from build123d import *

# Parameters (mm, degrees)
F1_DEPTH       = 110
F2_R           = 2
F4_D           = 8
F4_DEPTH       = 4
F6_D           = 4
F6_DEPTH       = 4
F6_CSINK_D     = 8
F6_CSINK_ANGLE = 90
F7_W           = 30
F7_H           = 13
F8_DEPTH       = 1


with BuildPart() as f1:
    # F0 (on Top) → F1 (new body)
    with BuildSketch(Plane.XY):
        Polygon((15, -18.36), (15, -15), (-15, -15), (-15, 15), (15, 15), (15, 18.36), (-18.36, 18.36), (-18.36, -18.36), align=None)
    extrude(amount=F1_DEPTH)

    # F2
    f2_edges = [f1.edges().sort_by_distance(p)[0] for p in [
        (-18.36, -18.36, 55),
        (-18.36, 18.36, 55),
        (15, -18.36, 55),
        (15, 18.36, 55),
    ]]
    fillet(f2_edges, radius=F2_R)

    # F4
    with Locations(Plane.XZ.offset(18.36)):
        with Locations((0, 30), (0, 80)):
            Hole(F4_D / 2, depth=F4_DEPTH)

    # F6
    with Locations(Plane.XZ.offset(-15)):
        with Locations((0, 30), (0, 80)):
            CounterSinkHole(F6_D / 2, F6_CSINK_D / 2, depth=F6_DEPTH, counter_sink_angle=F6_CSINK_ANGLE)

    # F7 (on face) → F8 (cut)
    with BuildSketch(Plane(origin=(0, -15, 0), x_dir=(-1, 0, 0), z_dir=(0, 1, 0))):
        with Locations((0, 96.5)):
            Rectangle(F7_W, F7_H)
    extrude(amount=-F8_DEPTH, mode=Mode.SUBTRACT)


solid = f1.part
The listing builds one solid part. Answer for the finished solid, in the listing's coordinates (mm). A direction names the side the tool comes from. Give positions to 0.01 mm unless a question says otherwise; leave off trailing zeros. Write each loop counter-clockwise with the first axis right and the second up, starting at its lowest first coordinate (ties: lowest second). Pieces come first, ordered by that corner, then holes.
1) A tool of negligible diameter and unlimited length cuts with its end or side. For faces 1 (the face through (0.521, -16.656, 33.966)), 2 (the face through (0, -15, 106)), 3 (the face through (-1, 18.36, 54)), from which of +Z, -Z, +X, -X, +Y, -Y can it reach the whole face along a straight path? Write none if from no direction.
2) Section D-D (y = 11) is taken. Write down the section's boundary in (x, z), and give its area (3 significant figures).
3) Given P1, Ø5, axis at x = 0, z = 30, coming from the +Y side; P2, Ø15.5, axis at y = -3.5, z = 70.5, coming from the +X side; P3, Ø5, axis at x = 0, z = 30, coming from the -Y side, each flat-ended and moving along its own axis, determine where each tip first touches the part or whether it passes through.
4) Section A-A (x = 6.5) is taken. Write down the section's boundary in (y, z), and give its area (3 significant figures).
5) Section B-B (z = 30) is taken. Write down the section's boundary in (x, y).
6) Find the intervals of material crossed by L1, parallel to Z at x = 0, y = 17.7; L2, parallel to Z at x = 0, y = -15.8; L3, parallel to Y at x = 1, z = 95, in increasing order.
7) For a pull along X with two mould halves and no side action, classify faces 4 (the face through (0, -16, 97)), 5 (the face through (0.867, -16.656, 76.095)), 6 (the face through (14.43, -17.76, 55.77)), 7 (the face through (0, 18, 82)) as pulls with the +X half, pulls with the -X half, needs draft (parallel to the pull), parting line crosses it, or undercut.
8) Section C-C (x = 0) is taken. Count the separate pieces of the cut face and the enclosed holes in it, and give its area (3 significant figures).
Response:
1. face 1: -Y
1. face 2: +Z, -Z, +X
1. face 3: +Z, -Z, +X, -X, +Y
2. outline: (-18.36, 0) - (-15, 0) - (-15, 110) - (-18.36, 110) - close
2. area: 370 mm2
3. P1: stops at y = 18.36
3. P2: stops at x = -15
3. P3: stops at y = 16.5
4. outline: (-18.36, 0) - (-15, 0) - (-15, 90) - (-16, 90) - (-16, 103) - (-15, 103) - (-15, 110) - (-18.36, 110) - close; (15, 0) - (18.36, 0) - (18.36, 110) - (15, 110) - close
4. area: 726 mm2
5. outline: (-18.36, -16.36) arc R2 ccw to (-16.36, -18.36) - (-4, -18.36) - (-4, -15) - (-15, -15) - (-15, 15) - (-4, 15) - (-2, 17) - (-2, 18.36) - (-16.36, 18.36) arc R2 ccw to (-18.36, 16.36) - close; (2, 17) - (4, 15) - (15, 15) - (15, 16.36) arc R2 ccw to (13, 18.36) - (2, 18.36) - close; (4, -18.36) - (13, -18.36) arc R2 ccw to (15, -16.36) - (15, -15) - (4, -15) - close
6. L1: z = 0 to 28, 32 to 78, 82 to 110
6. L2: z = 0 to 26, 34 to 76, 84 to 90, 103 to 110
6. L3: y = -18.36 to -16, 15 to 18.36
7. face 4: needs draft
7. face 5: undercut
7. face 6: pulls with the +X half
7. face 7: undercut
8. separate pieces: 6
8. enclosed holes: 0
8. area: 638 mm2
